For this review, take the finished solid that the model builds, in its own axes (mm). A direction names the side the tool comes from. Give positions to 0.01 mm unless a question says otherwise; leave off trailing zeros. Loops run counter-clockwise (first coordinate to the right, second up) from the corner with the lowest first, then second, coordinate; pieces in that order, holes last.
```python
from build123d import *

# Parameters (mm, degrees)
SKETCH10_R          = 4.5
BOSS_EXTRUDE6_DEPTH = 1.75
SKETCH13_R          = 1.8
BOSS_EXTRUDE7_DEPTH = 1.75
FILLET1_R           = 4
CUT_EXTRUDE2_DEPTH  = 1.5
SKETCH16_R          = 3
CUT_EXTRUDE3_DEPTH  = 1
CHAMFER1_SIZE       = 0.5
FILLET2_R           = 0.4


with BuildPart() as part:
    # Sketch10 → Boss-Extrude6 (new, symmetric)
    with BuildSketch(Plane.XY):
        with BuildLine():
            Line((-13.266499161, -7), (13.266499161, -7))
            ThreePointArc((13.266499161, -7), (0, 15), (-13.266499161, -7))
        make_face()
        Circle(SKETCH10_R, mode=Mode.SUBTRACT)
    extrude(amount=BOSS_EXTRUDE6_DEPTH, both=True)

    # Sketch13 → Boss-Extrude7 (add, symmetric)
    # profile 1 of 2: a face of its own
    with BuildSketch(Plane.XY):
        with BuildLine():
            Line((-4.3, 14.370455803), (-4.3, 19.1))
            ThreePointArc((-4.3, 19.1), (-3.421320344, 21.221320344), (-1.3, 22.1))
            Line((-1.3, 22.1), (1.3, 22.1))
            ThreePointArc((1.3, 22.1), (3.421320344, 21.221320344), (4.3, 19.1))
            Line((4.3, 19.1), (4.3, 14.370455803))
            ThreePointArc((4.3, 14.370455803), (0, 15), (-4.3, 14.370455803))
        make_face()
        with Locations((0, 17.8)):
            Circle(SKETCH13_R, mode=Mode.SUBTRACT)
    # profile 2 of 2: a face of its own
    with BuildSketch(Plane.XY):
        with BuildLine():
            Line((-14.59517979, 3.461318665), (-18.691085212, 5.826090764))
            ThreePointArc((-18.691085212, 5.826090764), (-20.088862691, 7.64770984), (-19.789161424, 9.924166975))
            Line((-19.789161424, 9.924166975), (-18.489161424, 12.175833025))
            ThreePointArc((-18.489161424, 12.175833025), (-16.667542348, 13.573610504), (-14.391085212, 13.273909236))
            Line((-14.391085212, 13.273909236), (-10.29517979, 10.909137138))
            ThreePointArc((-10.29517979, 10.909137138), (-12.990381057, 7.5), (-14.59517979, 3.461318665))
        make_face()
        with Locations((-15.415252187, 8.9)):
            Circle(SKETCH13_R, mode=Mode.SUBTRACT)
    extrude(amount=BOSS_EXTRUDE7_DEPTH, both=True)

    # Fillet1
    fillet1_edges = [part.edges().sort_by_distance(p)[0] for p in [
        (-4.3, 14.370455803, 0),
        (4.3, 14.370455803, 0),
        (-14.59517979, 3.461318665, 0),
        (-10.29517979, 10.909137138, 0),
        (13.266499161, -7, 0),
        (-13.266499161, -7, 0),
    ]]
    fillet(fillet1_edges, radius=FILLET1_R)

    # Sketch15 → Cut-Extrude2 (cut)
    with BuildSketch(Plane(origin=(0, 0, -1.75), x_dir=(-1, 0, 0), z_dir=(0, 0, -1))):
        with BuildLine():
            Line((-3.711309131, 8.453153894), (-7.336540279, 6.762680847))
            ThreePointArc((-7.336540279, 6.762680847), (-7.595077459, 6.480537025), (-7.578385042, 6.098217822))
            Line((-7.578385042, 6.098217822), (-6.944457649, 4.738756142))
            ThreePointArc((-6.944457649, 4.738756142), (-6.662313827, 4.480218962), (-6.279994625, 4.496911379))
            Line((-6.279994625, 4.496911379), (-2.654763477, 6.187384426))
            ThreePointArc((-2.654763477, 6.187384426), (-2.396226297, 6.469528248), (-2.412918714, 6.85184745))
            Line((-2.412918714, 6.85184745), (-3.046846106, 8.211309131))
            ThreePointArc((-3.046846106, 8.211309131), (-3.328989928, 8.46984631), (-3.711309131, 8.453153894))
        make_face()
        with BuildLine():
            Line((6.944457649, 4.738756142), (7.578385042, 6.098217822))
            ThreePointArc((7.578385042, 6.098217822), (7.595077459, 6.480537025), (7.336540279, 6.762680847))
            Line((7.336540279, 6.762680847), (3.711309131, 8.453153894))
            ThreePointArc((3.711309131, 8.453153894), (3.328989928, 8.46984631), (3.046846106, 8.211309131))
            Line((3.046846106, 8.211309131), (2.412918714, 6.85184745))
            ThreePointArc((2.412918714, 6.85184745), (2.396226297, 6.469528248), (2.654763477, 6.187384426))
            Line((2.654763477, 6.187384426), (6.279994625, 4.496911379))
            ThreePointArc((6.279994625, 4.496911379), (6.662313827, 4.480218962), (6.944457649, 4.738756142))
        make_face()
    extrude(amount=-CUT_EXTRUDE2_DEPTH, mode=Mode.SUBTRACT)

    # Sketch16 → Cut-Extrude3 (cut)
    with BuildSketch(Plane(origin=(0, 0, -1.75), x_dir=(-1, 0, 0), z_dir=(0, 0, -1))):
        with Locations((0, 17.8)):
            Circle(SKETCH16_R)
        with Locations((15.415252187, 8.9)):
            Circle(SKETCH16_R)
    extrude(amount=-CUT_EXTRUDE3_DEPTH, mode=Mode.SUBTRACT)

    # Chamfer1
    chamfer1_edges = [part.edges().sort_by_distance(p)[0] for p in [
        (3, 17.8, -1.75),
        (-12.415252187, 8.9, -1.75),
    ]]
    chamfer(chamfer1_edges, length=CHAMFER1_SIZE)

    # Fillet2
    fillet2_edges = [part.edges().sort_by_distance(p)[0] for p in [
        (3.421320344, 21.221320344, -1.75),
        (0, 22.1, -1.75),
        (-3.421320344, 21.221320344, -1.75),
        (-4.3, 18.09561291, -1.75),
        (-16.667542348, 13.573610504, -1.75),
        (-19.139161424, 11.05, -1.75),
        (-20.088862691, 7.64770984, -1.75),
        (-17.821260477, 5.323897219, -1.75),
        (-14.921492219, -1.5326676, -1.75),
        (4.3, 18.09561291, -1.75),
        (13.688725123, 6.133417032, -1.75),
        (-13.521260477, 12.771715691, -1.75),
        (-7.5, 12.990381057, -1.75),
        (0, -7, -1.75),
        (-12.995096001, -6.190896141, -1.75),
        (12.995096001, -6.190896141, -1.75),
        (-15.418049964, 3.232484708, -1.75),
        (4.909611108, 14.9686653, -1.75),
        (-10.508438857, 11.736180592, -1.75),
        (-4.909611108, 14.9686653, -1.75),
    ]]
    fillet(fillet2_edges, radius=FILLET2_R)


solid = part.part
```
Item 1: Take a section at C-C on z = 0.45. Give the boundary of the cut face in (x, y).
Answer:
outline: (-19.79, 9.92) arc R3 ccw to (-18.69, 5.83) - (-16.95, 4.82) arc R4 cw to (-14.96, 1.07) arc R15 ccw to (-14.43, -4.09) arc R4 ccw to (-10.58, -7) - (10.58, -7) arc R4 ccw to (14.43, -4.09) arc R15 ccw to (6.55, 13.49) arc R4 cw to (4.3, 17.09) - (4.3, 19.1) arc R3 ccw to (1.3, 22.1) - (-1.3, 22.1) arc R3 ccw to (-4.3, 19.1) - (-4.3, 17.09) arc R4 cw to (-6.55, 13.49) arc R15 ccw to (-8.41, 12.42) arc R4 cw to (-12.65, 12.27) - (-14.39, 13.27) arc R3 ccw to (-18.49, 12.18) - close; hole circle Ø3.6 at (-15.42, 8.9); hole circle Ø9 at (0, 0); hole circle Ø3.6 at (0, 17.8)
Item 2: Tool access review of faces 4 (the flat face through (-17.4, 8.9, -0.75)), 5 (the flat face through (-4.3, 18, 0)), 6 (the cylindrical face through (13.748, 5.999, 0.222)), 7 (the flat face through (4.3, 18, 0)), 8 (the flat face through (-13.533, 12.779, 0.222)): name each direction out of +Z, -Z, +X, -X, +Y, -Y from which nothing blocks a thin tool from reaching the whole face with its end or side.
Answer:
face 4: -Z
face 5: +Z, -Z, -X, +Y
face 6: +Z, -Z, +X
face 7: +Z, -Z, +X, +Y
face 8: +Z, -Z, +Y
Item 3: The part is to be moulded in two halves that separate along Y. For faces 1 (the flat face through (7.266, 5.428, -1.01)), 2 (the flat face through (1, 5, -1.75)), 3 (the flat face through (0, 22.1, 0)), say which applies: released by +Y, released by -Y, zero draft, split by the parting line, or undercut.
Answer:
face 1: undercut
face 2: zero draft
face 3: released by +Y
Item 4: Clearance check with flat-ended pins moving along their axes: pin 1 Ø0.6 at (y, z) = (17.5, -0.5) entering from -X; pin 2 Ø1.5 at (y, z) = (9.5, 1) entering from +X; pin 3 Ø1 at (y, z) = (10, 1) entering from -X. State where each tip first meets the part, or that it passes through.
Answer:
pin 1: stops at x = -4.3
pin 2: stops at x = 12.18
pin 3: stops at x = -19.99
Item 5: Take a section at A-A on y = 17.8. Give the boundary of the cut face in (x, z).
Answer:
outline: (-4.3, -1.35) arc R0.4 ccw to (-3.9, -1.75) - (-3.5, -1.75) - (-3, -1.25) - (-3, -0.75) - (-1.8, -0.75) - (-1.8, 1.75) - (-4.3, 1.75) - close; (1.8, -0.75) - (3, -0.75) - (3, -1.25) - (3.5, -1.75) - (3.9, -1.75) arc R0.4 ccw to (4.3, -1.35) - (4.3, 1.75) - (1.8, 1.75) - close
Item 6: For L1, parallel to Y at x = 0, z = -0.9; L2, parallel to Y at x = 0, z = -0.1; L3, parallel to X at y = 17.75, z = -1.1, list the stretches that pass through material, from the lowest coordinate up.
Answer:
L1: y = -7 to -4.5, 4.5 to 14.8, 20.8 to 22.1
L2: y = -7 to -4.5, 4.5 to 16, 19.6 to 22.1
L3: x = -4.3 to -3, 3 to 4.3
Item 7: Take a section at B-B on x = 0. Give the boundary of the cut face in (y, z), and give its area (3 significant figures).
Answer:
outline: (-7, -1.35) arc R0.4 ccw to (-6.6, -1.75) - (-4.5, -1.75) - (-4.5, 1.75) - (-7, 1.75) - close; (4.5, -1.75) - (14.3, -1.75) - (14.8, -1.25) - (14.8, -0.75) - (16, -0.75) - (16, 1.75) - (4.5, 1.75) - close; (19.6, -0.75) - (20.8, -0.75) - (20.8, -1.25) - (21.3, -1.75) - (21.7, -1.75) arc R0.4 ccw to (22.1, -1.35) - (22.1, 1.75) - (19.6, 1.75) - close
area: 55.0 mm2
